from build123d import *

# Parameters (mm, degrees)
SKETCH1_W           = 34.62
SKETCH1_H           = 42.12
SKETCH1_W_2         = 27
SKETCH1_H_2         = 34.5
BOSS_EXTRUDE1_DEPTH = 12
SKETCH2_W           = 5.75
SKETCH2_H           = 7.5
SKETCH2_R           = 1.25
BOSS_EXTRUDE2_DEPTH = 12
SKETCH3_W           = 15.5
SKETCH3_H           = 3.81
CUT_EXTRUDE1_DEPTH  = 30.785226204


with BuildPart() as part:
    # Sketch1 → Boss-Extrude1 (new body)
    with BuildSketch(Plane.XY):
        Rectangle(SKETCH1_W, SKETCH1_H)
        Rectangle(SKETCH1_W_2, SKETCH1_H_2, mode=Mode.SUBTRACT)
    extrude(amount=BOSS_EXTRUDE1_DEPTH)

    # Sketch2 → Boss-Extrude2 (add, through all)
    # profile 1 of 4: a face of its own
    with BuildSketch(Plane(origin=(0, 0, 0), x_dir=(-1, 0, 0), z_dir=(0, 0, -1))):
        with Locations((-10.625, 13.5)):
            Rectangle(SKETCH2_W, SKETCH2_H)
        with Locations((-10, 12.5)):
            Circle(SKETCH2_R, mode=Mode.SUBTRACT)
    # profile 2 of 4: a face of its own
    with BuildSketch(Plane(origin=(0, 0, 0), x_dir=(-1, 0, 0), z_dir=(0, 0, -1))):
        with Locations((10.625, 13.5)):
            Rectangle(SKETCH2_W, SKETCH2_H)
        with Locations(Location((10, 12.5, 0), (0, 0, 180))):
            Circle(SKETCH2_R, mode=Mode.SUBTRACT)
    # profile 3 of 4: a face of its own
    with BuildSketch(Plane(origin=(0, 0, 0), x_dir=(-1, 0, 0), z_dir=(0, 0, -1))):
        with Locations((10.625, -13.5)):
            Rectangle(SKETCH2_W, SKETCH2_H)
        with Locations((10, -12.5)):
            Circle(SKETCH2_R, mode=Mode.SUBTRACT)
    # profile 4 of 4: a face of its own
    with BuildSketch(Plane(origin=(0, 0, 0), x_dir=(-1, 0, 0), z_dir=(0, 0, -1))):
        with Locations((-10.625, -13.5)):
            Rectangle(SKETCH2_W, SKETCH2_H)
        with Locations(Location((-10, -12.5, 0), (0, 0, 180))):
            Circle(SKETCH2_R, mode=Mode.SUBTRACT)
    extrude(amount=-BOSS_EXTRUDE2_DEPTH)

    # Sketch3 → Cut-Extrude1 (cut, through all)
    with BuildSketch(Plane(origin=(0, 0, 0), x_dir=(-1, 0, 0), z_dir=(0, 0, -1))):
        with Locations((0, 19.155)):
            Rectangle(SKETCH3_W, SKETCH3_H)
    extrude(amount=-CUT_EXTRUDE1_DEPTH, mode=Mode.SUBTRACT)


solid = part.part
Part model, mm, in its own coordinate system. A direction names the side the tool comes from. Give positions to 0.01 mm unless a question says otherwise; leave off trailing zeros. Loops run counter-clockwise (first coordinate to the right, second up) from the corner with the lowest first, then second, coordinate; pieces in that order, holes last. Notation, with made-up numbers: M -21.75,81.5 L 3.25,81.5 A12 cw 3.25,85.5 Z; hole C 62,-10.75 d10. An arc over 180 degrees is marked long. Put each result on its own line as item: value. Start each with the question number.
1) Saw through at C-C (z = 10.5). List the corners of the cut face in (x, y), then the cut area to 3 significant figures.
2) Flat gauge pins, fed straight in: pin 1 (2 mm diameter, centred on x = 10, y = 12.5, fed in from -Z); pin 2 (3 mm diameter, centred on x = 2.5, y = -16, fed in from +Z). Where does each tip first touch, or does it go through?
3) Pull direction X, two halves, no side cores. Call faces 4 (the flat face through (-13, 21.06, 6)), 5 (the flat face through (7.75, 15, 6)), 6 (the flat face through (11, -9.75, 6)): +X half, -X half, draft (parallel to the pull), parting line (faces both ways), or undercut.
4) Probe probe 1 along Y at (x, z) = (-10, 7.5); probe 2 along X at (y, z) = (-8, 2.75); probe 3 along Y at (x, z) = (-12, 2.5). List the from-to ranges inside material, lowest first.
5) Saw through at A-A (y = 3). List the corners of the cut face in (x, z), then the cut area to 3 significant figures.
6) 3-axis set-ups, long thin cutter, end or side, ignore diameter. For faces 1 (the flat face through (-13.5, 0, 6)), 2 (the flat face through (0, -21.06, 6)), 3 (the flat face through (-7.75, -14, 6)): which of +Z, -Z, +X, -X, +Y, -Y reach the whole face in a straight line?
7) Saw through at B-B (x = 12.5). List the corners of the cut face in (y, z), then the cut area to 3 significant figures.
8) Saw through at D-D (y = -12.5). List the corners of the cut face in (x, z), then the cut area to 3 significant figures.
Numbers:
1. outline: M -17.31,-21.06 L 17.31,-21.06 L 17.31,21.06 L 7.75,21.06 L 7.75,9.75 L 13.5,9.75 L 13.5,-9.75 L 7.75,-9.75 L 7.75,-17.25 L -7.75,-17.25 L -7.75,-9.75 L -13.5,-9.75 L -13.5,9.75 L -7.75,9.75 L -7.75,21.06 L -17.31,21.06 Z; hole C -10,-12.5 d2.5; hole C -10,12.5 d2.5; hole C 10,-12.5 d2.5; hole C 10,12.5 d2.5
1. area: 621 mm^2
2. pin 1: through
2. pin 2: z = 12
3. face 4: draft
3. face 5: undercut
3. face 6: undercut
4. probe 1: -21.06 to -13.75, -11.25 to -9.75, 9.75 to 11.25, 13.75 to 21.06
4. probe 2: -17.31 to -13.5, 13.5 to 17.31
4. probe 3: -21.06 to -9.75, 9.75 to 21.06
5. outline: M -17.31,0 L -13.5,0 L -13.5,12 L -17.31,12 Z; M 13.5,0 L 17.31,0 L 17.31,12 L 13.5,12 Z
5. area: 91.4 mm^2
6. face 1: +Z, -Z
6. face 2: +Z, -Z, +X, -X, -Y
6. face 3: +Z, -Z, +Y
7. outline: M -21.06,0 L -9.75,0 L -9.75,12 L -21.06,12 Z; M 9.75,0 L 21.06,0 L 21.06,12 L 9.75,12 Z
7. area: 271 mm^2
8. outline: M -17.31,0 L -11.25,0 L -11.25,12 L -17.31,12 Z; M -8.75,0 L -7.75,0 L -7.75,12 L -8.75,12 Z; M 7.75,0 L 8.75,0 L 8.75,12 L 7.75,12 Z; M 11.25,0 L 17.31,0 L 17.31,12 L 11.25,12 Z
8. area: 169 mm^2
